Can you work these out from the model? Positions are in its coordinate system, mm. Face numbers are marked on the shaded views. A direction names the side the tool comes from. Give positions to 0.01 mm unless a question says otherwise; leave off trailing zeros. Order: outer loops, then holes, each group sorted by start corner. A loop starts at its lowest first (then second) coordinate and runs counter-clockwise, first axis right, second up. Notation, with made-up numbers: (-4.5, -29.5) - (9.5, -29.5) arc R23 ccw to (9.5, -2.5) - close; hole circle Ø6 at (6, 45.5). An arc over 180 degrees is marked (long way). Return JSON: item names as keys, results as strings.
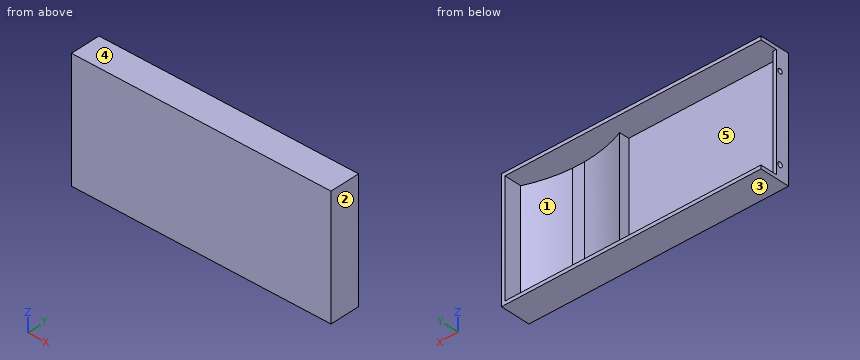
```python
from build123d import *

# Parameters (mm, degrees)
CROQUIS1_W              = 260
CROQUIS1_H              = 120
SALIENTE_EXTRUIR1_DEPTH = 30
VACIADO1_T              = -3.5
SALIENTE_EXTRUIR2_DEPTH = 113
CROQUIS3_W              = 113
CROQUIS3_H              = 24.257897879
CORTAR_EXTRUIR1_DEPTH   = 50.8
CROQUIS4_R              = 2.503701387
CROQUIS4_R_2            = 2.336787961
CORTAR_EXTRUIR2_DEPTH   = 50.8


# Read off the part's stored shape, not the designer's step: Saliente-Extruir2
with BuildPart() as part:
    # Croquis1 → Saliente-Extruir1 (new body)
    with BuildSketch(Plane(origin=(0, 0, 0), x_dir=(1, 0, 0), z_dir=(0, 1, 0))):
        Rectangle(CROQUIS1_W, CROQUIS1_H)
    extrude(amount=SALIENTE_EXTRUIR1_DEPTH)

    # Vaciado1
    vaciado1_openings = [part.faces().sort_by_distance(p)[0] for p in [
        (0, 30, 0),
    ]]
    offset(amount=VACIADO1_T, openings=vaciado1_openings, kind=Kind.INTERSECTION)

    # Saliente-Extruir2 outline → Saliente-Extruir2 (add)
    with BuildSketch(Plane.XY.offset(-56.5)):
        with BuildLine():
            Line((26.853568464, 3.5), (71.197774885, 3.5))
            ThreePointArc((71.197774885, 3.5), (48.599276947, 6.511555282), (26.853568464, 13.358871314))
            Line((26.853568464, 13.358871314), (26.853568464, 3.5))
        make_face()
        with BuildLine():
            ThreePointArc((126.5, 12.846828341), (105.349686421, 6.365747469), (83.415063898, 3.5))
            Line((83.415063898, 3.5), (126.5, 3.5))
            Line((126.5, 3.5), (126.5, 12.846828341))
        make_face()
    extrude(amount=SALIENTE_EXTRUIR2_DEPTH)

    # Croquis3 → Cortar-Extruir1 (cut)
    with BuildSketch(Plane.ZY.offset(130)):
        with Locations((0, 25.487820254)):
            Rectangle(CROQUIS3_W, CROQUIS3_H)
    extrude(amount=-CORTAR_EXTRUIR1_DEPTH, mode=Mode.SUBTRACT)

    # Croquis4 → Cortar-Extruir2 (cut)
    with BuildSketch(Plane.ZY.offset(130)):
        with Locations((-45.483908525, 9.241486811)):
            Circle(CROQUIS4_R)
        with Locations((38.97428492, 9.241486811)):
            Circle(CROQUIS4_R_2)
    extrude(amount=-CORTAR_EXTRUIR2_DEPTH, mode=Mode.SUBTRACT)


solid = part.part
```
1. Suppose I cut it at C-C (x = -3.5). List the corners of the cut face in (y, z) for me, plus the area to 4 significant figures.
Checks:
{"outline": "(0, -60) - (30, -60) - (30, -56.5) - (3.5, -56.5) - (3.5, 56.5) - (30, 56.5) - (30, 60) - (0, 60) - close", "area": "605.5 mm^2"}
2. Thinking about a two-plate mould opening in Z: for the marked faces 3, 4 and 5, which applies, +Z half, -Z half, draft (parallel to the pull), parting line (faces both ways), or undercut?
Checks:
{"face 3": "-Z half", "face 4": "+Z half", "face 5": "undercut"}
3. If I drill on L1, parallel to Z at x = -63.5, y = 24; L2, parallel to X at y = 28, z = -2.5; L3, parallel to Y at x = -118.5, z = 47, over which ranges is the centre line in solid material (lowest first)? Write a range as [from, to].
Checks:
{"L1": "[-60, -56.5], [56.5, 60]", "L2": "[126.5, 130]", "L3": "[0, 3.5]"}
4. On a 3-axis mill with a long thin cutter (end or side, diameter ignored), from which of +Z, -Z, +X, -X, +Y, -Y can I reach the whole of each face in a straight line? I mean the marked faces 1 and 2. Say none if no direction works.
Checks:
{"face 1": "+Y", "face 2": "+Z, -Z, +X, +Y, -Y"}
5. Suppose I cut it at A-A (z = -29). List the corners of the cut face in (x, y) for me, plus the area to 3 significant figures.
Checks:
{"outline": "(-130, 0) - (130, 0) - (130, 30) - (126.5, 30) - (126.5, 12.85) arc R132.27 cw to (83.42, 3.5) - (71.2, 3.5) arc R132.27 cw to (26.85, 13.36) - (26.85, 3.5) - (-126.5, 3.5) - (-126.5, 13.36) - (-130, 13.36) - close", "area": "1,340 mm^2"}
6. For pin 1 Ø6 at (x, z) = (-28.5, 17.5) entering from -Y; pin 2 Ø1.5 at (y, z) = (21, 24.5) entering from -X; pin 3 Ø1 at (x, z) = (-128, 11.5) entering from +Y; pin 4 Ø3 at (y, z) = (9.24, 38.97) entering from -X, each with a flat end and sliding along its axis, tell me the tip position at first contact or that it passes through.
Checks:
{"pin 1": "y = 0", "pin 2": "x = 126.5", "pin 3": "y = 13.36", "pin 4": "x = 26.85"}
7. Suppose I cut it at B-B (y = 18). List the corners of the cut face in (x, z) for me, plus the area to 3 significant figures.
Checks:
{"outline": "(-130, -60) - (130, -60) - (130, 60) - (-130, 60) - (-130, 56.5) - (126.5, 56.5) - (126.5, -56.5) - (-130, -56.5) - close", "area": "2,220 mm^2"}
